For this review, take the finished solid that the model builds, in its own axes (mm). A direction names the side the tool comes from. Round coordinates to 2 decimals unless told otherwise and drop trailing zeros. Order: outer loops, then holes, each group sorted by start corner. A loop starts at its lowest first (then second) coordinate and runs counter-clockwise, first axis right, second up. Notation, with made-up numbers: (50.25, -37.75) -> (54.25, -37.75) arc R20 ccw to (54.25, -8.75) -> close; hole circle Ø9 at (-35.75, 75.5). An arc over 180 degrees is marked (long way). Use a Markdown table: item, result. Add a question column.
1) Wall thickness on line 1 along X through (y, z) = (0.45, 65.2); line 2 along Z through (x, y) = (3, 1.3); line 3 along X through (y, z) = (1.05, 3.5): over which ranges is each line inside the solid? List them lowest first. Write a range as [from, to].
2) Draft analysis for pull direction Z (two halves, no side actions). For faces 1 (the face through (7, 1, 80)), 2 (the face through (3.75, 1.01, 7.03)), 3 (the face through (-12.5, 1, 70)), 4 (the face through (20.454, 1.014, 64.468)), state which applies: pulls with the +Z half, pulls with the -Z half, needs draft (parallel to the pull), parting line crosses it, or undercut.
3) Consider section D-D (z = 65.2). State the section outline as (x, y) points, plus the area to 3 significant figures.
4) Clearance check with flat-ended pins moving along their axes: P1, Ø0.6, axis at y = 1, z = 42.5, coming from the -X side; P2, Ø0.9, axis at x = 12, z = 7, coming from the +Y side. State where each tip first meets the part, or that it passes through.
5) Machinability: for faces 5 (the face through (7, 1, 0)), 6 (the face through (-6, 1, 60)), 7 (the face through (21, 1, 60)), which of the approach directions +Z, -Z, +X, -X, +Y, -Y give a long, thin tool a straight path to every point of the face, cutting with its end or side? Answer none if there is none.
6) Consider section A-A (z = 7). State the section outline as (x, y) points, plus the area to 3 significant figures.
7) Consider section C-C (y = 0.8). State the section outline as (x, z) points, plus the area to 3 significant figures.
8) Consider section B-B (x = 12). State the section outline as (y, z) points, plus the area to 3 significant figures.
```python
from build123d import *

# Parameters (mm, degrees)
SKETCH1_W           = 15
SKETCH1_H           = 2
BOSS_EXTRUDE1_DEPTH = 80
SKETCH2_W           = 40
SKETCH2_H           = 20
BOSS_EXTRUDE2_DEPTH = 2
SKETCH3_R           = 0.75
CUT_EXTRUDE1_DEPTH  = 85.618260441


with BuildPart() as part:
    # Sketch1 → Boss-Extrude1 (new body)
    with BuildSketch(Plane.XY):
        with Locations((7.5, 1)):
            Rectangle(SKETCH1_W, SKETCH1_H)
    extrude(amount=BOSS_EXTRUDE1_DEPTH)

    # Sketch2 → Boss-Extrude2 (add)
    with BuildSketch(Plane(origin=(0, 2, 0), x_dir=(1, 0, 0), z_dir=(0, 1, 0))):
        with Locations((7.5, -70)):
            Rectangle(SKETCH2_W, SKETCH2_H)
    extrude(amount=-BOSS_EXTRUDE2_DEPTH)

    # Sketch3 → Cut-Extrude1 (cut, through all)
    with BuildSketch(Plane(origin=(0, 2, 0), x_dir=(1, 0, 0), z_dir=(0, 1, 0))):
        with Locations(Location((20.291432582, -65.2, 0), (0, 0, 180))):
            Circle(SKETCH3_R)
        with Locations(Location((-8.208567418, -65.2, 0), (0, 0, 180))):
            Circle(SKETCH3_R)
        with Locations(Location((12, -7, 0), (0, 0, 180))):
            Circle(SKETCH3_R)
        with Locations(Location((3, -7, 0), (0, 0, 180))):
            Circle(SKETCH3_R)
    extrude(amount=-CUT_EXTRUDE1_DEPTH, mode=Mode.SUBTRACT)


solid = part.part
```
Results list:
| question | item | result |
|---|---|---|
| 1 | line 1 | [-12.5, -8.96], [-7.46, 19.54], [21.04, 27.5] |
| 1 | line 2 | [0, 6.25], [7.75, 80] |
| 1 | line 3 | [0, 15] |
| 2 | face 1 | pulls with the +Z half |
| 2 | face 2 | undercut |
| 2 | face 3 | needs draft |
| 2 | face 4 | undercut |
| 3 | outline | (-12.5, 0) -> (-8.96, 0) -> (-8.96, 2) -> (-12.5, 2) -> close; (-7.46, 0) -> (19.54, 0) -> (19.54, 2) -> (-7.46, 2) -> close; (21.04, 0) -> (27.5, 0) -> (27.5, 2) -> (21.04, 2) -> close |
| 3 | area | 74.0 mm2 |
| 4 | P1 | x = 0 |
| 4 | P2 | through |
| 5 | face 5 | -Z, +X, -X, +Y, -Y |
| 5 | face 6 | -Z, -X, +Y, -Y |
| 5 | face 7 | -Z, +X, +Y, -Y |
| 6 | outline | (0, 0) -> (2.25, 0) -> (2.25, 2) -> (0, 2) -> close; (3.75, 0) -> (11.25, 0) -> (11.25, 2) -> (3.75, 2) -> close; (12.75, 0) -> (15, 0) -> (15, 2) -> (12.75, 2) -> close |
| 6 | area | 24.0 mm2 |
| 7 | outline | (-12.5, 60) -> (0, 60) -> (0, 0) -> (15, 0) -> (15, 60) -> (27.5, 60) -> (27.5, 80) -> (-12.5, 80) -> close; hole circle Ø1.5 at (-8.21, 65.2); hole circle Ø1.5 at (3, 7); hole circle Ø1.5 at (12, 7); hole circle Ø1.5 at (20.29, 65.2) |
| 7 | area | 1,690 mm2 |
| 8 | outline | (0, 0) -> (2, 0) -> (2, 6.25) -> (0, 6.25) -> close; (0, 7.75) -> (2, 7.75) -> (2, 80) -> (0, 80) -> close |
| 8 | area | 157 mm2 |
